Check sheet for the modelled part. Datum: model origin and axes. Units: mm. Round coordinates to 2 decimals unless told otherwise and drop trailing zeros. Write each loop counter-clockwise with the first axis right and the second up, starting at its lowest first coordinate (ties: lowest second). Pieces come first, ordered by that corner, then holes. Notation, with made-up numbers: (-24, 26) -> (-18, 26) arc R19 ccw to (-18, 44) -> close; hole circle Ø8 at (51, -1.5). An arc over 180 degrees is marked (long way). Use one line per item in the form item = value. Start each with the question number.
```python
from build123d import *

# Parameters (mm, degrees)
BASE_FLANGE1_DEPTH = 1.2


# Sheet-metal steps are written as plain solids
with BuildPart() as part:
    # Sketch1 → Base-Flange1 (new body)
    with BuildSketch(Plane(origin=(0, 0, 0), x_dir=(1, 0, 0), z_dir=(0, 1, 0))):
        with BuildLine():
            Line((-455, -53), (455, -53))
            Line((455, -53), (455, -13))
            Line((455, -13), (495, -13))
            Line((495, -13), (495, -12))
            ThreePointArc((495, -12), (475.961940777, 33.961940777), (430, 53))
            Line((430, 53), (-430, 53))
            ThreePointArc((-430, 53), (-475.961940777, 33.961940777), (-495, -12))
            Line((-495, -12), (-495, -13))
            Line((-495, -13), (-455, -13))
            Line((-455, -13), (-455, -53))
        make_face()
    extrude(amount=-BASE_FLANGE1_DEPTH)


solid = part.part
```
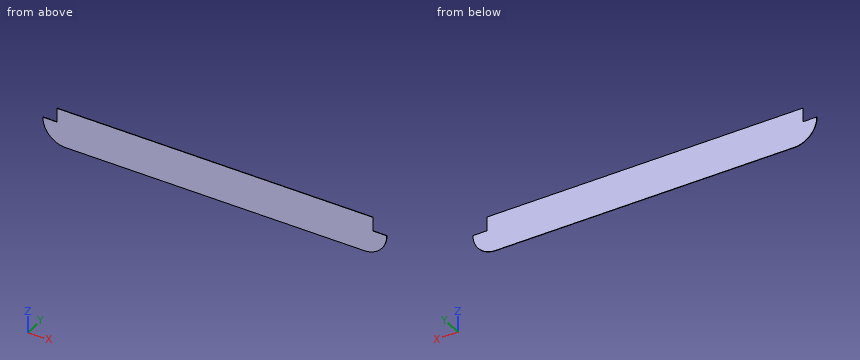
1. Sectioned sample at A-A (y = -0.9). Enter the section's corners in (x, z).
2. Scan lines: probe 1 along X at (y, z) = (-0.3, 45); probe 2 along X at (y, z) = (-0.45, 7.5); probe 3 along Z at (x, y) = (-437.5, -0.5). Record each from-to range of solid material in increasing order.
3. Sectioned sample at B-B (z = 28). Enter the section's corners in (x, y), and give its area (3 significant figures).
4. Sectioned sample at C-C (z = -35). Enter the section's corners in (x, y).
5. Depth check by flat-ended pin: pin 1 (0.6 mm diameter, centred on x = 471.5, y = -0.5, fed in from +Z); pin 2 (0.6 mm diameter, centred on y = -1, z = 31.5, fed in from -X). Enter the tip coordinate at first touch or a pass-through.
Returned:
q1.outline = (-495, 12) arc R65 ccw to (-430, -53) -> (430, -53) arc R65 ccw to (495, 12) -> (495, 13) -> (455, 13) -> (455, 53) -> (-455, 53) -> (-455, 13) -> (-495, 13) -> close
q2.probe_1 = -455 to 455
q2.probe_2 = -494.84 to 494.84
q2.probe_3 = -52.57 to 53
q3.outline = (-455, -1.2) -> (455, -1.2) -> (455, 0) -> (-455, 0) -> close
q3.area = 1,090 mm^2
q4.outline = (-474.9, -1.2) -> (474.9, -1.2) -> (474.9, 0) -> (-474.9, 0) -> close
q5.pin_1 = 13
q5.pin_2 = -455
